Source: CAD feature listing. Evaluate the final solid. Frame: model axes, mm. Face numbers are marked on the shaded views. A direction names the side the tool comes from. Give positions to 0.01 mm unless a question says otherwise; leave off trailing zeros. Write each loop counter-clockwise with the first axis right and the second up, starting at its lowest first coordinate (ties: lowest second). Pieces come first, ordered by that corner, then holes.
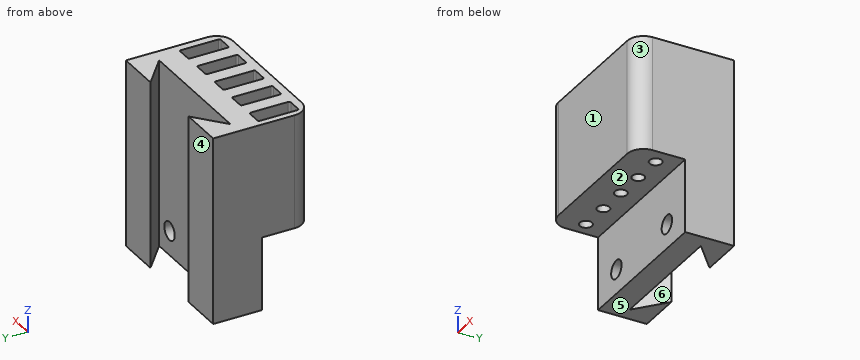
```python
from build123d import *

# Parameters (mm, degrees)
BOSS_EXTRUDE2_DEPTH = 25.4
SKETCH3_W           = 24.13
SKETCH3_H           = 17.78
BOSS_EXTRUDE3_DEPTH = 7.62
CUT_EXTRUDE2_DEPTH  = 16.51
SKETCH5_R           = 0.9525
CUT_EXTRUDE3_DEPTH  = 1.27
FILLET1_R           = 2.54
BOSS_EXTRUDE4_DEPTH = 3.81
SKETCH2_R           = 1.4351
CUT_EXTRUDE1_DEPTH  = 3.683


with BuildPart() as part:
    # Sketch1 → Boss-Extrude2 (new body)
    with BuildSketch(Plane.XY):
        Polygon((9.525, -21.59), (5.275147024, -21.59), (9.868313691, -25.527), (-9.868313691, -25.527), (-5.275147024, -21.59), (-9.525, -21.59), (-12.065, -21.59), (-12.065, -22.494104142), (-12.065, -29.21), (-8.343230433, -29.21), (10.89773699, -29.21), (12.065, -29.21), (12.065, -26.495103927), (12.065, -21.59), align=None)
    extrude(amount=BOSS_EXTRUDE2_DEPTH)

    # Sketch3 → Boss-Extrude3 (add)
    with BuildSketch(Plane(origin=(0, -29.21, 0), x_dir=(-1, 0, 0), z_dir=(0, -1, 0))):
        with Locations((0, -16.51)):
            Rectangle(SKETCH3_W, SKETCH3_H)
    extrude(amount=BOSS_EXTRUDE3_DEPTH)

    # Sketch4 → Cut-Extrude2 (cut)
    with BuildSketch(Plane.XY.offset(25.4)):
        with BuildLine():
            Line((10.541, -35.56), (8.509, -35.56))
            ThreePointArc((8.509, -35.56), (8.329394878, -35.485605122), (8.255, -35.306))
            Line((8.255, -35.306), (8.255, -29.464))
            ThreePointArc((8.255, -29.464), (8.329394878, -29.284394878), (8.509, -29.21))
            Line((8.509, -29.21), (10.541, -29.21))
            ThreePointArc((10.541, -29.21), (10.720605122, -29.284394878), (10.795, -29.464))
            Line((10.795, -29.464), (10.795, -35.306))
            ThreePointArc((10.795, -35.306), (10.720605122, -35.485605122), (10.541, -35.56))
        make_face()
        with BuildLine():
            Line((5.969, -35.306), (5.969, -29.464))
            ThreePointArc((5.969, -29.464), (5.894605122, -29.284394878), (5.715, -29.21))
            Line((5.715, -29.21), (3.683, -29.21))
            ThreePointArc((3.683, -29.21), (3.503394878, -29.284394878), (3.429, -29.464))
            Line((3.429, -29.464), (3.429, -35.306))
            ThreePointArc((3.429, -35.306), (3.503394878, -35.485605122), (3.683, -35.56))
            Line((3.683, -35.56), (5.715, -35.56))
            ThreePointArc((5.715, -35.56), (5.894605122, -35.485605122), (5.969, -35.306))
        make_face()
        with BuildLine():
            Line((1.143, -35.306), (1.143, -29.464))
            ThreePointArc((1.143, -29.464), (1.068605122, -29.284394878), (0.889, -29.21))
            Line((0.889, -29.21), (-1.143, -29.21))
            ThreePointArc((-1.143, -29.21), (-1.322605122, -29.284394878), (-1.397, -29.464))
            Line((-1.397, -29.464), (-1.397, -35.306))
            ThreePointArc((-1.397, -35.306), (-1.322605122, -35.485605122), (-1.143, -35.56))
            Line((-1.143, -35.56), (0.889, -35.56))
            ThreePointArc((0.889, -35.56), (1.068605122, -35.485605122), (1.143, -35.306))
        make_face()
        with BuildLine():
            Line((-3.683, -35.306), (-3.683, -29.464))
            ThreePointArc((-3.683, -29.464), (-3.757394878, -29.284394878), (-3.937, -29.21))
            Line((-3.937, -29.21), (-5.969, -29.21))
            ThreePointArc((-5.969, -29.21), (-6.148605122, -29.284394878), (-6.223, -29.464))
            Line((-6.223, -29.464), (-6.223, -35.306))
            ThreePointArc((-6.223, -35.306), (-6.148605122, -35.485605122), (-5.969, -35.56))
            Line((-5.969, -35.56), (-3.937, -35.56))
            ThreePointArc((-3.937, -35.56), (-3.757394878, -35.485605122), (-3.683, -35.306))
        make_face()
        with BuildLine():
            Line((-8.509, -35.306), (-8.509, -29.464))
            ThreePointArc((-8.509, -29.464), (-8.583394878, -29.284394878), (-8.763, -29.21))
            Line((-8.763, -29.21), (-10.795, -29.21))
            ThreePointArc((-10.795, -29.21), (-10.974605122, -29.284394878), (-11.049, -29.464))
            Line((-11.049, -29.464), (-11.049, -35.306))
            ThreePointArc((-11.049, -35.306), (-10.974605122, -35.485605122), (-10.795, -35.56))
            Line((-10.795, -35.56), (-8.763, -35.56))
            ThreePointArc((-8.763, -35.56), (-8.583394878, -35.485605122), (-8.509, -35.306))
        make_face()
    extrude(amount=-CUT_EXTRUDE2_DEPTH, mode=Mode.SUBTRACT)

    # Sketch5 → Cut-Extrude3 (cut)
    with BuildSketch(Plane.XY.offset(8.89)):
        with Locations((9.525, -32.385)):
            Circle(SKETCH5_R)
        with Locations((4.699, -32.385)):
            Circle(SKETCH5_R)
        with Locations((-0.127, -32.385)):
            Circle(SKETCH5_R)
        with Locations((-4.953, -32.385)):
            Circle(SKETCH5_R)
        with Locations((-9.779, -32.385)):
            Circle(SKETCH5_R)
    extrude(amount=-CUT_EXTRUDE3_DEPTH, mode=Mode.SUBTRACT)

    # Fillet1
    fillet1_edges = [part.edges().sort_by_distance(p)[0] for p in [
        (12.065, -36.83, 16.51),
        (-12.065, -36.83, 16.51),
    ]]
    fillet(fillet1_edges, radius=FILLET1_R)

    # Sketch6 → Boss-Extrude4 (add)
    with BuildSketch(Plane(origin=(0, 0, 0), x_dir=(-1, 0, 0), z_dir=(0, 0, -1))):
        Polygon((-12.065, -29.21), (12.065, -29.21), (12.065, -21.59), (5.275147024, -21.59), (9.868313691, -25.527), (-9.868313691, -25.527), (-5.275147024, -21.59), (-12.065, -21.59), align=None)
    extrude(amount=BOSS_EXTRUDE4_DEPTH)

    # Sketch2 → Cut-Extrude1 (cut)
    with BuildSketch(Plane(origin=(0, -29.21, 0), x_dir=(-1, 0, 0), z_dir=(0, -1, 0))):
        with Locations(Location((-6.985, 0, 0), (0, 0, 90))):
            Circle(SKETCH2_R)
        with Locations(Location((6.985, 0, 0), (0, 0, 90))):
            Circle(SKETCH2_R)
    extrude(amount=-CUT_EXTRUDE1_DEPTH, mode=Mode.SUBTRACT)


solid = part.part
```
1. Line query: L1, parallel to X at y = -31.75, z = 21.25 (3 decimals); L2, parallel to X at y = -26.35, z = 0 (3 decimals); L3, parallel to Y at x = 9.25, z = 14. Output: solid intervals per line, ascending.
2. Cut plane B-B, the plane y = -33.75. Return the cut outline in (x, z) (3 decimals).
3. Access query for the marked faces 1 and 2. Directions: +Z, -Z, +X, -X, +Y, -Y. A direction counts if a zero-diameter tool reaches every point of the face in a straight line with its end or side. Return the directions, or none.
4. Cut plane A-A, the plane z = 0. Return the cut outline in (x, y) (3 decimals), then the cut area to 3 significant figures.
5. Cut plane D-D, the plane y = -22.75. Return the cut outline in (x, z) (3 decimals), then the cut area to 3 significant figures.
6. Contact query for flat-ended pins moving along their axis: P1, Ø1, axis at x = 0, z = 14, coming from the +Y side; P2, Ø3, axis at y = -35, z = 4.5, coming from the -X side; P3, Ø2, axis at x = 9.5, y = -32.5, coming from the +Z side; P4, Ø5, axis at x = 3, y = -35, coming from the -Z side. Output: stop coordinate, or through.
7. Cut plane C-C, the plane x = 4.5. Return the cut outline in (y, z), then the cut area to 3 significant figures.
8. Mould query, pull axis Y, two halves, no side actions, for the marked faces 3, 4, 5 and 6. Classes: +Y half, -Y half, draft (parallel to the pull), parting line (faces both ways), or undercut.
Response values:
1. L1: x = -12.065 to -11.049, -8.509 to -6.223, -3.683 to -1.397, 1.143 to 3.429, 5.969 to 8.255, 10.795 to 12.065
1. L2: x = -12.065 to -8.42, -5.55 to 5.55, 8.42 to 12.065
1. L3: y = -36.83 to -35.56, -29.21 to -25.53, -25 to -21.59
2. outline: (-12.065, 7.62) - (12.065, 7.62) - (12.065, 25.4) - (10.795, 25.4) - (10.795, 8.89) - (8.255, 8.89) - (8.255, 25.4) - (5.969, 25.4) - (5.969, 8.89) - (3.429, 8.89) - (3.429, 25.4) - (1.143, 25.4) - (1.143, 8.89) - (-1.397, 8.89) - (-1.397, 25.4) - (-3.683, 25.4) - (-3.683, 8.89) - (-6.223, 8.89) - (-6.223, 25.4) - (-8.509, 25.4) - (-8.509, 8.89) - (-11.049, 8.89) - (-11.049, 25.4) - (-12.065, 25.4) - close
3. face 1: +Z, -Z, +X, -X, -Y
3. face 2: -Z, +X, -X, -Y
4. outline: (-12.065, -29.21) - (-8.42, -29.21) - (-8.42, -25.527) - (-9.868, -25.527) - (-5.275, -21.59) - (-12.065, -21.59) - close; (-5.55, -29.21) - (5.55, -29.21) - (5.55, -25.527) - (-5.55, -25.527) - close; (5.275, -21.59) - (9.868, -25.527) - (8.42, -25.527) - (8.42, -29.21) - (12.065, -29.21) - (12.065, -21.59) - close
4. area: 103 mm2
5. outline: (-12.065, -3.81) - (-6.628, -3.81) - (-6.628, 25.4) - (-12.065, 25.4) - close; (6.628, -3.81) - (12.065, -3.81) - (12.065, 25.4) - (6.628, 25.4) - close
5. area: 318 mm2
6. P1: stops at y = -25.53
6. P2: passes through
6. P3: stops at z = 8.89
6. P4: stops at z = 7.62
7. outline: (-36.83, 7.62) - (-33.32, 7.62) - (-33.32, 8.89) - (-35.56, 8.89) - (-35.56, 25.4) - (-36.83, 25.4) - close; (-31.45, 7.62) - (-29.21, 7.62) - (-29.21, -3.81) - (-25.53, -3.81) - (-25.53, 25.4) - (-29.21, 25.4) - (-29.21, 8.89) - (-31.45, 8.89) - close
7. area: 136 mm2
8. face 3: -Y half
8. face 4: +Y half
8. face 5: draft
8. face 6: undercut
